CAD build for the part. Positions are in the model's coordinates, mm. A direction names the side the tool comes from. Give positions to 0.01 mm unless a question says otherwise; leave off trailing zeros. Loops run counter-clockwise (first coordinate to the right, second up) from the corner with the lowest first, then second, coordinate; pieces in that order, holes last. Notation, with made-up numbers: M -16.5,60 L 40.5,60 A17 ccw 40.5,83 Z; hole C 86.25,0.5 d1. An arc over 180 degrees is marked long. Answer as CSV lines item,"result".
from build123d import *

# Parameters (mm, degrees)
SKETCH1_R           = 2
BOSS_EXTRUDE1_DEPTH = 7


with BuildPart() as part:
    # Sketch1 → Boss-Extrude1 (new body)
    with BuildSketch(Plane(origin=(0, 0, 0), x_dir=(1, 0, 0), z_dir=(0, 1, 0))):
        with BuildLine():
            Line((13.032630063, 87.579564679), (13.867369937, 87.579564679))
            Line((13.867369937, 87.579564679), (26.9, 12))
            ThreePointArc((26.9, 12), (18.414718626, -8.485281374), (38.9, 0))
            Line((38.9, 0), (18.45, 90))
            Line((18.45, 90), (13.45, 90))
            Line((13.45, 90), (8.45, 90))
            Line((8.45, 90), (-12, 0))
            ThreePointArc((-12, 0), (8.485281374, -8.485281374), (0, 12))
            Line((0, 12), (13.032630063, 87.579564679))
        make_face()
        with Locations(Location((0, 0, 0), (0, 0, 270))):
            Circle(SKETCH1_R, mode=Mode.SUBTRACT)
        with Locations(Location((26.9, 0, 0), (0, 0, 270))):
            Circle(SKETCH1_R, mode=Mode.SUBTRACT)
    extrude(amount=BOSS_EXTRUDE1_DEPTH)


solid = part.part
1) Which spindle directions (+Z, -Z, +X, -X, +Y, -Y) get a long thin tool onto all of the face, cutting with end or side? Do faces 1 (the face through (20.292, 3.451, -50.319)), 2 (the face through (14, 3, -90)). Say none if no direction does.
Answer below:
face 1,"+Y, -Y"
face 2,"-Z, +X, -X, +Y, -Y"
2) Band-saw the part on A-A on y = 4.25. Give the cut face in (x, z).
Answer below:
outline,"M -12,0 L 8.45,-90 L 18.45,-90 L 38.9,0 A12 ccw long 26.9,-12 L 13.87,-87.58 L 13.03,-87.58 L 0,-12 A12 ccw long Z; hole C 0,0 d4; hole C 26.9,0 d4"
3) Mould opens along Z. For faces 3 (the face through (28.82, 3.45, -44.37)), 4 (the face through (24.948, 3.451, -0.434)), 5 (the face through (24.4, 7, -28.4)) say: +Z half, -Z half, draft (parallel to the pull), parting line (faces both ways), or undercut.
Answer below:
face 3,"-Z half"
face 4,"undercut"
face 5,"draft"
4) Band-saw the part on C-C on x = 4. Give the cut face in (y, z), and give its area (3 significant figures).
Answer below:
outline,"M 0,-70.42 L 7,-70.42 L 7,-35.2 L 0,-35.2 Z; M 0,-11.31 L 7,-11.31 L 7,11.31 L 0,11.31 Z"
area,"405 mm^2"
5) Band-saw the part on B-B on z = -78.5. Give the cut face in (x, y), and give its area (3 significant figures).
Answer below:
outline,"M 5.84,0 L 11.47,0 L 11.47,7 L 5.84,7 Z; M 15.43,0 L 21.06,0 L 21.06,7 L 15.43,7 Z"
area,"78.8 mm^2"
6) Drill centre lines: line 1 (X direction, y = 4, z = -28.5); line 2 (X direction, y = 1.25, z = -64). Where is each one in solid material? Low to high. Write a range as from..to.
Answer below:
line 1,"x = -5.52..2.85, 24.05..32.42"
line 2,"x = 2.54..8.97, 17.93..24.36"
7) Flat gauge pins, fed straight in: pin 1 (3.5 mm diameter, centred on x = 26.9, z = 0, fed in from -Y); pin 2 (1.5 mm diameter, centred on y = 5, z = -75.5, fed in from -X); pin 3 (4 mm diameter, centred on y = 4, z = -17, fed in from +X); pin 4 (1.5 mm diameter, centred on y = 6, z = -62, fed in from +X). Where does each tip first touch, or does it go through?
Answer below:
pin 1,"passes through"
pin 2,"stops at x = 4.98"
pin 3,"stops at x = 35.49"
pin 4,"stops at x = 24.98"
